Here's how the part is built. I have some questions about the finished solid (model axes, mm). Face numbers are marked on the shaded views. A direction names the side the tool comes from. Round coordinates to 2 decimals unless told otherwise and drop trailing zeros. Write each loop counter-clockwise with the first axis right and the second up, starting at its lowest first coordinate (ties: lowest second). Pieces come first, ordered by that corner, then holes. Notation, with made-up numbers: (17.5, -30) -> (26.5, -30) arc R22 cw to (26.5, 3) -> close; hole circle Ø9 at (17, 59.5). An arc over 180 degrees is marked (long way). Put each result on its own line as item: value. Start each with the question number.
1) I want a section at B-B, the plane y = 43. List the corners of the cut face in (x, z) for me, then the cut area to 3 significant figures.
2) I want a section at A-A, the plane z = 36. List the corners of the cut face in (x, y) for me, then the cut area to 3 significant figures.
3) I want a section at C-C, the plane x = -2. List the corners of the cut face in (y, z) for me.
4) I want a section at D-D, the plane z = 26. List the corners of the cut face in (x, y) for me.
5) Will these pins go through, and if not, where does the flat tip stop? P1, Ø7.5, axis at x = 0.5, y = 12.5, coming from the +Z side; P2, Ø1, axis at x = 11, z = 8, coming from the -Y side; P3, Ø5, axis at y = 4.5, z = 36, coming from the -X side; P4, Ø11, axis at y = 48.3, z = -12.94, coming from the -X side.
6) We'd pull the mould along Z, two halves only. Please class the marked faces 3, 4 and 5: released by +Z, released by -Z, zero draft, split by the parting line, or undercut.
7) If I drill on line 1 along X through (y, z) = (26, 24); line 2 along Y through (x, z) = (-13.5, 29.5); line 3 along Y through (x, z) = (13.75, -6.5), over which ranges is the centre line in solid material (lowest first)? Write a range as [from, to].
8) Which directions (+Z, -Z, +X, -X, +Y, -Y) give clear straight access to the entire face, cutting with the end or side of a thin tool? Please do the marked faces 1 and 2.
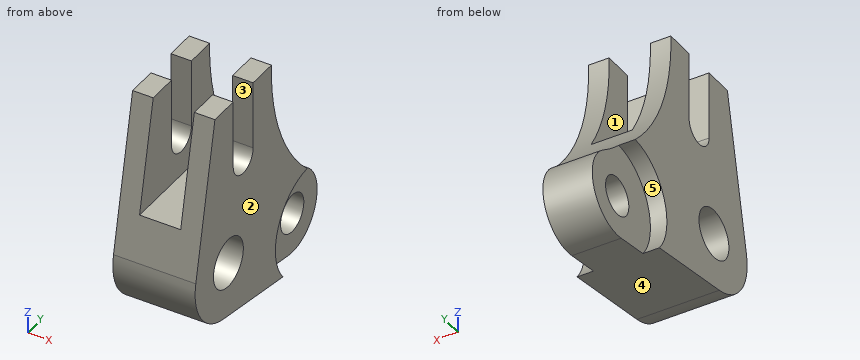
from build123d import *

# Parameters (mm, degrees)
IZIM2_R                     = 7
IZIM2_R_2                   = 9
Y_KSEKLIK_EKSTR_ZYON1_DEPTH = 15
IZIM3_R                     = 20
KES_EKSTR_ZYON1_DEPTH       = 6
KES_EKSTR_ZYON4_DEPTH       = 18
KES_EKSTR_ZYON4_DEPTH_BACK  = 77.999207989
IZIM5_W                     = 15
IZIM5_H                     = 40


with BuildPart() as part:
    # Çizim2 → Yükseklik-Ekstrüzyon1 (new, symmetric)
    with BuildSketch(Plane(origin=(0, 0, 0), x_dir=(0, 0, -1), z_dir=(1, 0, 0))):
        with BuildLine():
            Line((19.739319337, -3.218582315), (27.745441758, 45.882354578))
            ThreePointArc((27.745441758, 45.882354578), (18.474216993, 62.238421042), (0.510195975, 56.691307592))
            ThreePointArc((0.510195975, 56.691307592), (-25.763963339, 33.475550855), (-60, 25.912707322))
            Line((-60, 25.912707322), (-60, 14.912707322))
            Line((-60, 14.912707322), (-35, 14.912707322))
            ThreePointArc((-35, 14.912707322), (-29, 8.912707322), (-35, 2.912707322))
            Line((-35, 2.912707322), (-60, 2.912707322))
            Line((-60, 2.912707322), (-60, -8.087292678))
            Line((-60, -8.087292678), (-4.01109025, -19.593650885))
            ThreePointArc((-4.01109025, -19.593650885), (11.352533428, -16.465721508), (19.739319337, -3.218582315))
        make_face()
        with Locations((12.940952255, 48.296291314)):
            Circle(IZIM2_R, mode=Mode.SUBTRACT)
        Circle(IZIM2_R_2, mode=Mode.SUBTRACT)
    extrude(amount=Y_KSEKLIK_EKSTR_ZYON1_DEPTH, both=True)

    # Çizim3 → Kes-Ekstrüzyon1 (cut)
    with BuildSketch(Plane(origin=(15, 0, 0), x_dir=(0, 0, -1), z_dir=(1, 0, 0))):
        with Locations((12.940952255, 48.296291314)):
            Circle(IZIM3_R)
    kes_ekstr_zyon1 = extrude(amount=-KES_EKSTR_ZYON1_DEPTH, mode=Mode.SUBTRACT)

    # Aynalama1: Kes-Ekstrüzyon1 across plane
    add(kes_ekstr_zyon1.mirror(Plane(origin=(0, 0, 0), x_dir=(0, 0, 1), z_dir=(1, 0, 0))), mode=Mode.SUBTRACT)

    # Çizim5 → Kes-Ekstrüzyon4 (cut, two sides: drawn at the far end of the back side and taken through both)
    with BuildSketch(Plane(origin=(0, 25.86805022, 0), x_dir=(1, 0, 0), z_dir=(0, 1, 0)).offset(-KES_EKSTR_ZYON4_DEPTH_BACK)):
        with Locations((0.003643514, -40)):
            Rectangle(IZIM5_W, IZIM5_H)
    extrude(amount=KES_EKSTR_ZYON4_DEPTH + KES_EKSTR_ZYON4_DEPTH_BACK, mode=Mode.SUBTRACT)


solid = part.part
Findings:
1. outline: (-15, 6.35) -> (-9, 6.35) -> (-9, -8.36) -> (9, -8.36) -> (9, 6.35) -> (15, 6.35) -> (15, 11.62) -> (-15, 11.62) -> close; (-9, -27.28) -> (9, -27.28) -> (9, -17.52) -> (-9, -17.52) -> close
1. area: 599 mm2
2. outline: (-15, -13.02) -> (-7.5, -13.02) -> (-7.5, 2.91) -> (-15, 2.91) -> close; (-15, 14.91) -> (-7.5, 14.91) -> (-7.5, 29.25) -> (-15, 29.25) -> close; (7.5, -13.02) -> (15, -13.02) -> (15, 2.91) -> (7.5, 2.91) -> close; (7.5, 14.91) -> (15, 14.91) -> (15, 29.25) -> (7.5, 29.25) -> close
2. area: 454 mm2
3. outline: (-19.59, 4.01) arc R20 ccw to (-3.22, -19.74) -> (45.88, -27.75) arc R15 ccw to (56.69, -0.51) arc R70 cw to (36.76, 20) -> (-16.31, 20) -> close; hole circle Ø18 at (0, 0); hole circle Ø14 at (48.3, -12.94)
4. outline: (-15, -15.07) -> (-7.5, -15.07) -> (-7.5, 33.36) -> (-15, 33.36) -> close; (7.5, -15.07) -> (15, -15.07) -> (15, 33.36) -> (7.5, 33.36) -> close
5. P1: stops at z = 20
5. P2: stops at y = -18.88
5. P3: stops at x = -15
5. P4: passes through
6. face 3: zero draft
6. face 4: released by -Z
6. face 5: undercut
7. line 1: x = [-15, -7.5], [7.5, 15]
7. line 2: y = [-14.36, 6.51], [11.31, 31.71]
7. line 3: y = [-18.91, -6.22], [6.22, 29.36]
8. face 1: +Z, +Y, -Y
8. face 2: +Z, -Z, +X, +Y, -Y
